```python
from build123d import *

# Parameters (mm, degrees)
F1_DEPTH = 1.5
F2_DEPTH = 3
F4_DEPTH = 3
F5_R     = 0.74999
F6_R     = 0.75


# Not quite as in the source:
# - a fillet or chamfer is up to 0.001 mm smaller than in the source, because OpenCascade refuses the exact size


with BuildPart() as f1:
    # F0 (on Front) → F1 (new body)
    with BuildSketch(Plane.XZ):
        with BuildLine():
            ThreePointArc((-19.05, -14.2875), (-17.6550960454, -17.6550960454), (-14.2875, -19.05))
            Line((-14.2875, -19.05), (14.2875, -19.05))
            ThreePointArc((14.2875, -19.05), (17.6550960454, -17.6550960454), (19.05, -14.2875))
            Line((19.05, -14.2875), (19.05, 14.2875))
            ThreePointArc((19.05, 14.2875), (17.6550960454, 17.6550960454), (14.2875, 19.05))
            Line((14.2875, 19.05), (-14.2875, 19.05))
            ThreePointArc((-14.2875, 19.05), (-17.6550960454, 17.6550960454), (-19.05, 14.2875))
            Line((-19.05, 14.2875), (-19.05, -14.2875))
        make_face()
        Polygon((15.791487975, -0.306085875), (0, -16.09757385), (-11.48107305, -4.616510325), (-8.829722625, -1.9651599), (0.16503015, -10.95990315), (4.083738975, -7.0411848), (2.315441775, -5.2728876), (4.9667922, -2.621537175), (6.735098925, -4.389834375), (10.65380775, -0.471116025), (1.6590645, 8.523627225), (4.310414925, 11.17497765), align=None, mode=Mode.SUBTRACT)
        Polygon((-6.975852825, 4.018416525), (-13.5459216, -2.55165225), (-16.09757385, 0), (-0.306085875, 15.791487975), (2.245566375, 13.239835725), (-4.3245024, 6.66976695), (3.025206675, -0.679942125), (0.37385625, -3.331302075), align=None, mode=Mode.SUBTRACT)
    extrude(amount=F1_DEPTH)

    # F0 (on Front) → F2 (join)
    with BuildSketch(Plane.XZ):
        Polygon((-16.09757385, 0), (-13.5459216, -2.55165225), (-6.975852825, 4.018416525), (0.37385625, -3.331302075), (3.025206675, -0.679942125), (-4.3245024, 6.66976695), (2.245566375, 13.239835725), (-0.306085875, 15.791487975), align=None)
        Polygon((-11.48107305, -4.616510325), (0, -16.09757385), (15.791487975, -0.306085875), (4.310414925, 11.17497765), (1.6590645, 8.523627225), (10.65380775, -0.471116025), (6.735098925, -4.389834375), (4.9667922, -2.621537175), (2.315441775, -5.2728876), (4.083738975, -7.0411848), (0.16503015, -10.95990315), (-8.829722625, -1.9651599), align=None)
    extrude(amount=F2_DEPTH)

    # F3 (on face) → F4 (join)
    with BuildSketch(Plane.XZ):
        with BuildLine():
            ThreePointArc((-14.2875, 19.05), (-17.6550960454, 17.6550960454), (-19.05, 14.2875))
            Line((-19.05, 14.2875), (-19.05, -14.2875))
            ThreePointArc((-19.05, -14.2875), (-17.6550960454, -17.6550960454), (-14.2875, -19.05))
            Line((-14.2875, -19.05), (14.2875, -19.05))
            ThreePointArc((14.2875, -19.05), (17.6550960454, -17.6550960454), (19.05, -14.2875))
            Line((19.05, -14.2875), (19.05, 14.2875))
            ThreePointArc((19.05, 14.2875), (17.6550960454, 17.6550960454), (14.2875, 19.05))
            Line((14.2875, 19.05), (-14.2875, 19.05))
        make_face()
        with BuildLine():
            ThreePointArc((-17.55, 14.2875), (-16.5944358736, 16.5944358736), (-14.2875, 17.55))
            Line((-14.2875, 17.55), (14.2875, 17.55))
            ThreePointArc((14.2875, 17.55), (16.5944358736, 16.5944358736), (17.55, 14.2875))
            Line((17.55, 14.2875), (17.55, -14.2875))
            ThreePointArc((17.55, -14.2875), (16.5944358736, -16.5944358736), (14.2875, -17.55))
            Line((14.2875, -17.55), (-14.2875, -17.55))
            ThreePointArc((-14.2875, -17.55), (-16.5944358736, -16.5944358736), (-17.55, -14.2875))
            Line((-17.55, -14.2875), (-17.55, 14.2875))
        make_face(mode=Mode.SUBTRACT)
    extrude(amount=F4_DEPTH)

    # F5 (radius 0.75 in the source; OpenCascade refuses exactly that, so slightly less here)
    f5_edges = [f1.edges().sort_by_distance(p)[0] for p in [
        (-4.332346, -3, -6.462532),
        (-10.155398, -3, -3.290835),
        (-5.740537, -3, -10.357042),
        (7.895744, -3, -8.20183),
        (10.050951, -3, 5.434446),
        (2.98474, -3, 9.849302),
        (6.156436, -3, 4.026256),
        (8.694453, -3, -2.430475),
        (5.850946, -3, -3.505686),
        (3.641117, -3, -3.947212),
        (3.19959, -3, -6.157036),
        (2.124385, -3, -9.000544),
        (-8.20183, -3, 7.895744),
        (-14.821748, -3, -1.275826),
        (-10.260887, -3, 0.733382),
        (-3.300998, -3, 0.343557),
        (1.699531, -3, -2.005622),
        (-0.649648, -3, 2.994912),
        (-1.039468, -3, 9.954801),
        (0.96974, -3, 14.515662),
        (-17.655096, -3, 17.655096),
        (-19.05, -3, 0),
        (-17.655096, -3, -17.655096),
        (0, -3, -19.05),
        (17.655096, -3, -17.655096),
        (19.05, -3, 0),
        (17.655096, -3, 17.655096),
        (0, -3, 19.05),
        (-16.594436, -3, 16.594436),
        (0, -3, 17.55),
        (16.594436, -3, 16.594436),
        (17.55, -3, 0),
        (16.594436, -3, -16.594436),
        (0, -3, -17.55),
        (-16.594436, -3, -16.594436),
        (-17.55, -3, 0),
    ]]
    fillet(f5_edges, radius=F5_R)

    # F6
    f6_edges = [f1.edges().sort_by_distance(p)[0] for p in [
        (-17.655096, 0, -17.655096),
        (0, 0, -19.05),
        (17.655096, 0, -17.655096),
        (19.05, 0, 0),
        (17.655096, 0, 17.655096),
        (0, 0, 19.05),
        (-17.655096, 0, 17.655096),
        (-19.05, 0, 0),
    ]]
    fillet(f6_edges, radius=F6_R)


solid = f1.part
```
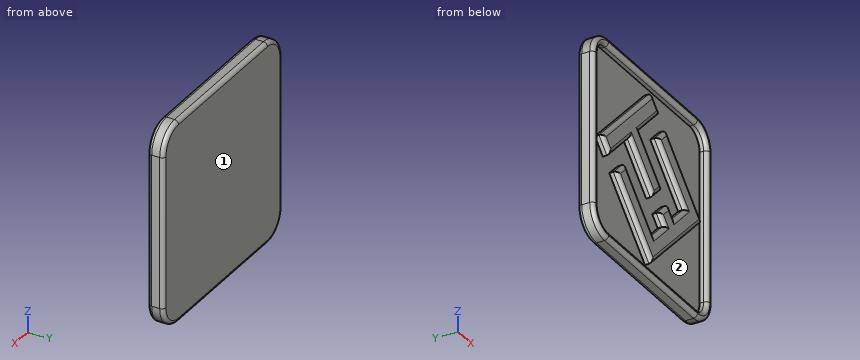
For this review, take the finished solid that the model builds, in its own axes (mm). Face numbers are marked on the shaded views. Coordinates: 2 decimals unless noted, no trailing zeros. Answer as CSV lines item,"result".
Q1. Clearance check with a flat-ended pin moving along its axis: pin 1 Ø1.5 at (x, z) = (-14, 13.5) entering from -Y. State where the tip first meets the part, or that it passes through.
Model answer:
pin 1,"stops at y = -1.5"
Q2. Wall thickness on line 1 along Z through (x, y) = (-11, -1.95); line 2 along Z through (x, y) = (-2.5, -2.6) (3 decimals); line 3 along X through (y, z) = (-2.4, 14): over which ranges is each line inside the solid? List them lowest first. Write a range as [from, to].
Model answer:
line 1,"z = [-19.05, -17.55], [-5.1, -4.14], [-0.01, 5.1], [17.55, 19.05]"
line 2,"z = [-18.963, -17.637], [-13.475, -8.417], [-0.335, 4.723], [8.617, 13.475], [17.637, 18.963]"
line 3,"x = [-19.03, -17.57], [-2.08, 1.46], [17.57, 19.03]"
Q3. Draft analysis for pull direction Z (two halves, no side actions). For the marked faces 1 and 2, state which applies: released by +Z, released by -Z, zero draft, split by the parting line, or undercut.
Model answer:
face 1,"zero draft"
face 2,"undercut"
